For this review, take the finished solid that the model builds, in its own axes (mm). A direction names the side the tool comes from. Coordinates: 2 decimals unless noted, no trailing zeros. Order: outer loops, then holes, each group sorted by start corner. A loop starts at its lowest first (then second) coordinate and runs counter-clockwise, first axis right, second up. Notation, with made-up numbers: (28.5, 35.5) -> (71.5, 35.5) arc R17 cw to (71.5, 47.5) -> close; hole circle Ø11 at (74.25, 4.25). An arc over 180 degrees is marked (long way). Write item = value, one per line. Start each with the question number.
1) Wall thickness on probe 1 along Y at (x, z) = (-79, 9) (3 decimals); probe 2 along Z at (x, y) = (-24, 4): over which ranges is each line inside the solid? List them lowest first. Write a range as [from, to].
2) Machinability: for faces 4 (the face through (-138, 16, 3.175)), 5 (the face through (-142, 3.175, 19)), 6 (the face through (-279.4, 2, 13)), 7 (the face through (7.03, 16.06, 5.49)), which of the approach directions +Z, -Z, +X, -X, +Y, -Y give a long, thin tool a straight path to every point of the face, cutting with its end or side? Answer none if there is none.
3) Consider section B-B on y = 16.5. Give the boundary of the cut face in (x, z) (3 decimals).
4) Consider section A-A on x = -25.4. Give the boundary of the cut face in (y, z) (3 decimals).
5) Draft analysis for pull direction X (two halves, no side actions). For faces 1 (the face through (-277.59, 1.61, 29.84)), 2 (the face through (3, 6.985, 3)), 3 (the face through (-286.43, 16.32, 5.49)), state which applies: +X half, -X half, draft (parallel to the pull), parting line (faces both ways), or undercut.
6) Insertion check: pin 1 Ø2.5 at (y, z) = (1.5, 20) entering from -X; pin 2 Ø8 at (x, z) = (-252.5, 15.5) entering from +Y (3 decimals); pin 3 Ø3.5 at (y, z) = (1.5, 19) entering from +X; pin 4 Ø1.5 at (x, z) = (-118.5, 24) entering from -Y. Each pin has a flat end and moves straight along its axis. Give the tip position at first contact, or say it passes through.
7) Consider section C-C on x = -240. Give the boundary of the cut face in (y, z) (3 decimals), and give its area (3 significant figures).
from build123d import *

# Parameters (mm, degrees)
SKETCH3_W                    = 279.4
SKETCH3_H                    = 31.75
BASE_FLANGE1_DEPTH           = 3.175
EDGE_FLANGE1_STRIP_W         = 20.32
EDGE_FLANGE1_STRIP_H         = 3.175
EDGE_FLANGE1_STRIP_CUT_DEPTH = 279.4
EDGE_FLANGE1_DEPTH           = 279.4
EDGE_FLANGE2_DEPTH           = 18.415
EDGE_FLANGE3_DEPTH           = 18.415
FILLET1_R                    = 6.35
O_0_316_DIAMETER_SLOT2_DEPTH = 3.175
O_0_316_DIAMETER_SLOT1_DEPTH = 3.175


# Read off the part's stored shape, not the designer's step: O (0.316) Diameter Slot2, O (0.316) Diameter Slot1
# Sheet-metal steps are written as plain solids
with BuildPart() as part:
    # Sketch3 → Base-Flange1 (new body)
    with BuildSketch(Plane(origin=(0, 0, 0), x_dir=(1, 0, 0), z_dir=(0, 1, 0))):
        with Locations((-139.7, -15.875)):
            Rectangle(SKETCH3_W, SKETCH3_H)
    extrude(amount=BASE_FLANGE1_DEPTH)

    # Edge-Flange1 strip (across the edge) → Edge-Flange1 strip cut (cut)
    with BuildSketch(Plane(origin=(0, 3.175, 0), x_dir=(0, 0, 1), z_dir=(-1, 0, 0))):
        with Locations((-3.175, -1.5875)):
            Rectangle(EDGE_FLANGE1_STRIP_W, EDGE_FLANGE1_STRIP_H)
    extrude(amount=EDGE_FLANGE1_STRIP_CUT_DEPTH, mode=Mode.SUBTRACT)

    # Edge-Flange1 section (across the edge) → Edge-Flange1 (add)
    with BuildSketch(Plane(origin=(0, 3.175, 0), x_dir=(0, 0, 1), z_dir=(-1, 0, 0))):
        with BuildLine():
            Line((0, 3.81), (0, 22.225))
            Line((0, 22.225), (3.175, 22.225))
            Line((3.175, 22.225), (3.175, 3.81))
            ThreePointArc((3.175, 3.81), (4.290923164, 1.115923164), (6.985, 0))
            Line((6.985, 0), (6.985, -3.175))
            ThreePointArc((6.985, -3.175), (2.045859133, -1.129140867), (0, 3.81))
        make_face()
    extrude(amount=EDGE_FLANGE1_DEPTH)

    # Edge-Flange2 section (across the edge) → Edge-Flange2 (add)
    with BuildSketch(Plane(origin=(0.671805796, 6.985, 3.175), x_dir=(-0.3420201433256631, 2.7658990361859502e-15, 0.9396926207859105), z_dir=(0, 1, 0))):
        with BuildLine():
            Line((-3.175, 0.671805796), (-3.175, 12.7))
            Line((-3.175, 12.7), (0, 12.7))
            Line((0, 12.7), (0, 0.671805796))
            ThreePointArc((0, 0.671805796), (0.057882461, 0.01020624), (0.229771115, -0.63129095))
            Line((0.229771115, -0.63129095), (-2.753752956, -1.717204905))
            ThreePointArc((-2.753752956, -1.717204905), (-3.068882155, -0.541126725), (-3.175, 0.671805796))
        make_face()
    extrude(amount=EDGE_FLANGE2_DEPTH)

    # Edge-Flange3 section (across the edge) → Edge-Flange3 (add)
    with BuildSketch(Plane(origin=(-280.071805796, 25.4, 3.175), x_dir=(0.3420201433256631, 1.2835487003775482e-15, 0.9396926207859105), z_dir=(0, -1, 0))):
        with BuildLine():
            Line((-3.175, 0.671805796), (-3.175, 12.7))
            Line((-3.175, 12.7), (0, 12.7))
            Line((0, 12.7), (0, 0.671805796))
            ThreePointArc((0, 0.671805796), (0.057882461, 0.01020624), (0.229771115, -0.63129095))
            Line((0.229771115, -0.63129095), (-2.753752956, -1.717204905))
            ThreePointArc((-2.753752956, -1.717204905), (-3.068882155, -0.541126725), (-3.175, 0.671805796))
        make_face()
    extrude(amount=EDGE_FLANGE3_DEPTH)

    # Fillet1
    fillet1_edges = [part.edges().sort_by_distance(p)[0] for p in [
        (13.148859058, 6.985, 6.026893785),
        (13.148859058, 25.4, 6.026893785),
        (-292.548859058, 25.4, 6.026893785),
        (-292.548859058, 6.985, 6.026893785),
        (0, 1.5875, 31.75),
        (-279.4, 1.5875, 31.75),
    ]]
    fillet(fillet1_edges, radius=FILLET1_R)

    # O (0.316) Diameter Slot2 outline → O (0.316) Diameter Slot2 (cut)
    with BuildSketch(Plane(origin=(0, 0, 0), x_dir=(1, 0, 0), z_dir=(0, 1, 0))):
        with BuildLine():
            Line((-29.4132, -16.7132), (-29.4132, -21.3868))
            ThreePointArc((-29.4132, -21.3868), (-25.4, -25.4), (-21.3868, -21.3868))
            Line((-21.3868, -21.3868), (-21.3868, -16.7132))
            ThreePointArc((-21.3868, -16.7132), (-25.4, -12.7), (-29.4132, -16.7132))
        make_face()
        with BuildLine():
            Line((-258.0132, -16.7132), (-258.0132, -21.3868))
            ThreePointArc((-258.0132, -21.3868), (-254, -25.4), (-249.9868, -21.3868))
            Line((-249.9868, -21.3868), (-249.9868, -16.7132))
            ThreePointArc((-249.9868, -16.7132), (-254, -12.7), (-258.0132, -16.7132))
        make_face()
    extrude(amount=O_0_316_DIAMETER_SLOT2_DEPTH, mode=Mode.SUBTRACT)

    # O (0.316) Diameter Slot1 outline → O (0.316) Diameter Slot1 (cut)
    with BuildSketch(Plane(origin=(0, 0, 0), x_dir=(1, 0, 0), z_dir=(0, 1, 0))):
        with BuildLine():
            Line((-16.7132, -15.1257), (-16.7132, -22.9743))
            ThreePointArc((-16.7132, -22.9743), (-12.7, -26.9875), (-8.6868, -22.9743))
            Line((-8.6868, -22.9743), (-8.6868, -15.1257))
            ThreePointArc((-8.6868, -15.1257), (-12.7, -11.1125), (-16.7132, -15.1257))
        make_face()
        with BuildLine():
            Line((-270.7132, -15.1257), (-270.7132, -22.9743))
            ThreePointArc((-270.7132, -22.9743), (-266.7, -26.9875), (-262.6868, -22.9743))
            Line((-262.6868, -22.9743), (-262.6868, -15.1257))
            ThreePointArc((-262.6868, -15.1257), (-266.7, -11.1125), (-270.7132, -15.1257))
        make_face()
    extrude(amount=O_0_316_DIAMETER_SLOT1_DEPTH, mode=Mode.SUBTRACT)


solid = part.part
Answer sheet:
q1.probe_1 = [0, 3.175]
q1.probe_2 = [0.67, 4.62]
q2.face_4 = +Z, +Y
q2.face_5 = +Z, +X, -X, +Y
q2.face_6 = +Z, -Z, -X, -Y
q2.face_7 = +Z, +Y, -Y
q3.outline = (-293.092, 4.535) -> (-281.789, 0.421) arc R6.985 ccw to (-279.4, 0) -> (0, 0) arc R6.985 ccw to (2.389, 0.421) -> (13.692, 4.535) -> (12.606, 7.519) -> (1.303, 3.405) arc R3.81 cw to (0, 3.175) -> (-279.4, 3.175) arc R3.81 cw to (-280.703, 3.405) -> (-292.006, 7.519) -> close
q4.outline = (0, 6.985) arc R6.985 ccw to (6.985, 0) -> (25.4, 0) -> (25.4, 3.175) -> (6.985, 3.175) arc R3.81 cw to (3.175, 6.985) -> (3.175, 12.7) -> (0, 12.7) -> close; (0, 25.4) -> (3.175, 25.4) -> (3.175, 31.75) -> (0, 31.75) -> close
q5.face_1 = -X half
q5.face_2 = draft
q5.face_3 = undercut
q6.pin_1 = -279.4
q6.pin_2 = 3.175
q6.pin_3 = 0
q6.pin_4 = 0
q7.outline = (0, 6.985) arc R6.985 ccw to (6.985, 0) -> (25.4, 0) -> (25.4, 3.175) -> (6.985, 3.175) arc R3.81 cw to (3.175, 6.985) -> (3.175, 31.75) -> (0, 31.75) -> close
q7.area = 164 mm2
